Model file for the job. Use its own axes, mm. A direction names the side the tool comes from. Round coordinates to 2 decimals unless told otherwise and drop trailing zeros. Loops run counter-clockwise (first coordinate to the right, second up) from the corner with the lowest first, then second, coordinate; pieces in that order, holes last. Notation, with made-up numbers: M 46.25,-23 L 94.25,-23 A22 cw 94.25,6 Z; hole C 3.25,31 d5. An arc over 180 degrees is marked long. Use a Markdown table: item, result. Add a question column.
Q1. Cut at B-B (x = 44.5). Give the cut face in (y, z) (3 decimals), plus the area to 3 significant figures.
Q2. Cut at D-D (z = -58). Give the cut face in (x, y), plus the area to 3 significant figures.
Q3. Probe line 1 (Y direction, x = 30, z = -24.5) (3 decimals); line 2 (Y direction, x = -8, z = 21); line 3 (Y direction, x = -56.5, z = 19). List the from-to ranges inside material, lowest first. Write a range as from..to.
Q4. Tool access for faces 4 (the face through (-11.012, 398.574, -49.592)), 5 (the face through (-19, 374.65, 20)), 6 (the face through (10.241, 336.372, -34.737)): list every direction of +Z, -Z, +X, -X, +Y, -Y with a clear straight run to the whole face (end or side of a thin tool).
Q5. Cut at A-A (z = 44). Give the cut face in (x, y) (3 decimals).
Q6. Pin check, flat tips, straight feed: pin 1 (4 mm diameter, centred on x = -28.5, y = 109.5, fed in from -Z); pin 2 (10 mm diameter, centred on x = 0, y = 129, fed in from -Z); pin 3 (20.5 mm diameter, centred on y = 363, z = -22, fed in from +X); pin 4 (12 mm diameter, centred on y = 191, z = 27.5, fed in from -X). Stop position of each tip, or through.
Q7. Mould opens along Y. For faces 1 (the face through (-5.506, 382.699, -24.796)), 2 (the face through (76.2, 95, 0)), 3 (the face through (-20, 31.75, 19)) say: +Y half, -Y half, draft (parallel to the pull), parting line (faces both ways), or undercut.
Q8. Cut at C-C (y = 164.5). Give the cut face in (x, z), plus the area to 3 significant figures.
from build123d import *

# Parameters (mm, degrees)
F5_R      = 50.8
F6_DEPTH  = 15.875
F7_R      = 50.8
F8_DEPTH  = 15.875
F9_R      = 19.05
F10_DEPTH = 25.4
F11_R     = 19.05
F12_DEPTH = 25.4
F13_R     = 19.05
F14_DEPTH = 25.4
F15_R     = 19.05
F16_DEPTH = 25.4
F17_W     = 50.8
F17_H     = 101.6
F18_DEPTH = 25.4
F19_W     = 50.8
F19_H     = 101.6
F20_DEPTH = 25.4
F21_W     = 101.6
F21_H     = 50.8
F22_DEPTH = 25.4
F23_W     = 101.6
F23_H     = 50.8
F24_DEPTH = 25.4
F25_W     = 50.8
F25_H     = 101.6
F26_DEPTH = 25.4
F27_W     = 50.8
F27_H     = 101.6
F28_DEPTH = 25.4
F29_W     = 101.6
F29_H     = 50.8
F30_DEPTH = 25.4
F31_W     = 101.6
F31_H     = 50.8
F32_DEPTH = 25.4
F33_R     = 25.4
F34_DEPTH = 15.875
F35_R     = 25.4
F36_DEPTH = 12.7
F37_R     = 25.4
F38_DEPTH = 12.7
F39_R     = 25.4
F40_DEPTH = 12.7
F41_R     = 25.4
F42_DEPTH = 15.875


with BuildPart() as f6:
    # F5 (on offset) → F6 (new body)
    with BuildSketch(Plane.XZ.offset(-406.4)):
        Circle(F5_R)
    extrude(amount=F6_DEPTH)



with BuildPart() as f8:
    # F7 (on Front) → F8 (new body)
    with BuildSketch(Plane.XZ):
        Circle(F7_R)
    extrude(amount=-F8_DEPTH)



with BuildPart() as f10:
    # F9 (on offset) → F10 (new body)
    with BuildSketch(Plane.XZ.offset(-57.15)):
        with Locations((50.8, 0)):
            Circle(F9_R)
    extrude(amount=-F10_DEPTH)

    # F29 (on face) → F30 (join)
    with BuildSketch(Plane.XZ.offset(-57.15)):
        with Locations((25.4, 0)):
            Rectangle(F29_W, F29_H)
    extrude(amount=F30_DEPTH)

    # F31 (on face) → F32 (join)
    with BuildSketch(Plane(origin=(0, 82.55, 0), x_dir=(-1, 0, 0), z_dir=(0, 1, 0))):
        with Locations((-25.4, 0)):
            Rectangle(F31_W, F31_H)
    extrude(amount=F32_DEPTH)


with BuildPart() as f12:
    # F11 (on offset) → F12 (new body)
    with BuildSketch(Plane.XZ.offset(-146.05)):
        with Locations((0, 50.8)):
            Circle(F11_R)
    extrude(amount=-F12_DEPTH)

    # F25 (on face) → F26 (join)
    with BuildSketch(Plane.XZ.offset(-146.05)):
        with Locations((0, 25.4)):
            Rectangle(F25_W, F25_H)
    extrude(amount=F26_DEPTH)

    # F27 (on face) → F28 (join)
    with BuildSketch(Plane(origin=(0, 171.45, 0), x_dir=(-1, 0, 0), z_dir=(0, 1, 0))):
        with Locations((0, 25.4)):
            Rectangle(F27_W, F27_H)
    extrude(amount=F28_DEPTH)


with BuildPart() as f14:
    # F13 (on offset) → F14 (new body)
    with BuildSketch(Plane.XZ.offset(-234.95)):
        with Locations((-50.8, 0)):
            Circle(F13_R)
    extrude(amount=-F14_DEPTH)

    # F21 (on face) → F22 (join)
    with BuildSketch(Plane.XZ.offset(-234.95)):
        with Locations((-25.4, 0)):
            Rectangle(F21_W, F21_H)
    extrude(amount=F22_DEPTH)

    # F23 (on face) → F24 (join)
    with BuildSketch(Plane(origin=(0, 260.35, 0), x_dir=(-1, 0, 0), z_dir=(0, 1, 0))):
        with Locations((25.4, 0)):
            Rectangle(F23_W, F23_H)
    extrude(amount=F24_DEPTH)


with BuildPart() as f16:
    # F15 (on offset) → F16 (new body)
    with BuildSketch(Plane.XZ.offset(-323.85)):
        with Locations((0, -50.8)):
            Circle(F15_R)
    extrude(amount=-F16_DEPTH)

    # F17 (on face) → F18 (join)
    with BuildSketch(Plane.XZ.offset(-323.85)):
        with Locations((0, -25.4)):
            Rectangle(F17_W, F17_H)
    extrude(amount=F18_DEPTH)

    # F19 (on face) → F20 (join)
    with BuildSketch(Plane(origin=(0, 349.25, 0), x_dir=(-1, 0, 0), z_dir=(0, 1, 0))):
        with Locations((0, -25.4)):
            Rectangle(F19_W, F19_H)
    extrude(amount=F20_DEPTH)


with BuildPart() as f8_1:
    add(f8.part)

    add(f10.part)  # F34 merges F10
    # F33 (on face) → F34 (join, through all)
    with BuildSketch(Plane(origin=(0, 15.875, 0), x_dir=(-1, 0, 0), z_dir=(0, 1, 0))):
        Circle(F33_R)
    extrude(amount=F34_DEPTH)


    add(f12.part)  # F36 merges F12
    # F35 (on face) → F36 (join, through all)
    with BuildSketch(Plane.XZ.offset(-120.65)):
        Circle(F35_R)
    extrude(amount=F36_DEPTH)


    add(f14.part)  # F38 merges F14
    # F37 (on face) → F38 (join, through all)
    with BuildSketch(Plane.XZ.offset(-209.55)):
        Circle(F37_R)
    extrude(amount=F38_DEPTH)


    add(f16.part)  # F40 merges F16
    # F39 (on face) → F40 (join, through all)
    with BuildSketch(Plane.XZ.offset(-298.45)):
        Circle(F39_R)
    extrude(amount=F40_DEPTH)


with BuildPart() as f6_1:
    add(f6.part)

    add(f8_1.part)  # F42 merges F8
    # F41 (on face) → F42 (join, through all)
    with BuildSketch(Plane.XZ.offset(-390.525)):
        Circle(F41_R)
    extrude(amount=F42_DEPTH)


solid = f6_1.part
Checked values:
| question | item | result |
|---|---|---|
| 1 | outline | M 0,-24.503 L 15.875,-24.503 L 15.875,24.503 L 0,24.503 Z; M 31.75,-25.4 L 57.15,-25.4 L 57.15,-17.978 L 82.55,-17.978 L 82.55,-25.4 L 107.95,-25.4 L 107.95,25.4 L 82.55,25.4 L 82.55,17.978 L 57.15,17.978 L 57.15,25.4 L 31.75,25.4 Z; M 390.525,-24.503 L 406.4,-24.503 L 406.4,24.503 L 390.525,24.503 Z |
| 1 | area | 5,050 mm^2 |
| 2 | outline | M -25.4,298.45 L 25.4,298.45 L 25.4,323.85 L 17.64,323.85 L 17.64,349.25 L 25.4,349.25 L 25.4,374.65 L -25.4,374.65 L -25.4,349.25 L -17.64,349.25 L -17.64,323.85 L -25.4,323.85 Z |
| 2 | area | 3,480 mm^2 |
| 3 | line 1 | y = 0..15.875, 31.75..57.15, 82.55..107.95, 390.525..406.4 |
| 3 | line 2 | y = 0..57.15, 82.55..146.05, 171.45..234.95, 260.35..323.85, 349.25..406.4 |
| 3 | line 3 | y = 209.55..234.95, 260.35..285.75 |
| 4 | face 4 | +Y |
| 4 | face 5 | +Z, -X |
| 4 | face 6 | none |
| 5 | outline | M -25.4,120.65 L 25.4,120.65 L 25.4,146.05 L 17.795,146.05 L 17.795,171.45 L 25.4,171.45 L 25.4,196.85 L -25.4,196.85 L -25.4,171.45 L -17.795,171.45 L -17.795,146.05 L -25.4,146.05 Z; M -25.39,0 L 25.39,0 L 25.39,15.875 L -25.39,15.875 Z; M -25.39,390.525 L 25.39,390.525 L 25.39,406.4 L -25.39,406.4 Z |
| 6 | pin 1 | passes through |
| 6 | pin 2 | stops at z = -25.4 |
| 6 | pin 3 | stops at x = 25.4 |
| 6 | pin 4 | stops at x = -25.4 |
| 7 | face 1 | undercut |
| 7 | face 2 | draft |
| 7 | face 3 | undercut |
| 8 | outline | C 0,50.8 d38.1 |
| 8 | area | 1,140 mm^2 |
